Answer from the drawing. Dimensions are ordinates in mm from the lowest x, y and z of the part. A direction names the side the tool comes from. Coordinates: 2 decimals unless noted, no trailing zeros. Order: outer loops, then holes, each group sorted by start corner. A loop starts at its lowest first (then second) coordinate and runs counter-clockwise, first axis right, second up. Notation, with made-up numbers: (24.25, 87.5) -> (77.25, 87.5) arc R13 ccw to (77.25, 108.5) -> close; hole circle Ø2 at (20, -2). An arc over 180 degrees is marked (long way). Answer in a Markdown table with one row per item.
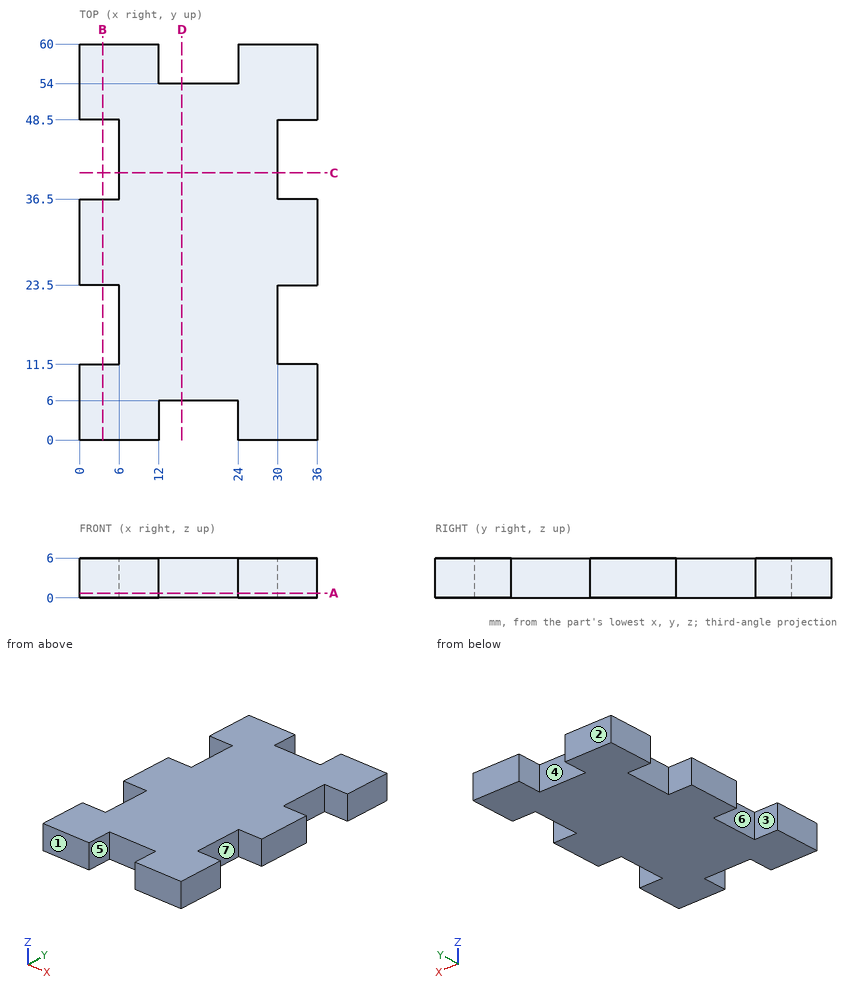
(1) Which of the six approach directions +Z, -Z, +X, -X, +Y, -Y give full straight-line access (tool end or side, diameter ignored) to the marked faces 4, 5, 6 and 7?
Check values:
| item | result |
|---|---|
| face 4 | +Z, -Z, +Y |
| face 5 | +Z, -Z, -Y |
| face 6 | +Z, -Z, -X |
| face 7 | +Z, -Z, +X |
(2) Find the intervals of material crossed by line 1 along Y through (x, z) = (31, 4.05); line 2 along X through (y, z) = (57, 1.9); line 3 along Y through (x, z) = (14, 3.95), in increasing order. Write a range as from..to.
Check values:
| item | result |
|---|---|
| line 1 | 0..11.5, 23.5..36.5, 48.5..60 |
| line 2 | 0..12, 24..36 |
| line 3 | 6..54 |
(3) A cutting plane is placed at A-A, the plane z = 0.7. Determine the outline of the cut face in (x, y).
Check values:
| item | result |
|---|---|
| outline | (0, 0) -> (12, 0) -> (12, 6) -> (24, 6) -> (24, 0) -> (36, 0) -> (36, 11.5) -> (30, 11.5) -> (30, 23.5) -> (36, 23.5) -> (36, 36.5) -> (30, 36.5) -> (30, 48.5) -> (36, 48.5) -> (36, 60) -> (24, 60) -> (24, 54) -> (12, 54) -> (12, 60) -> (0, 60) -> (0, 48.5) -> (6, 48.5) -> (6, 36.5) -> (0, 36.5) -> (0, 23.5) -> (6, 23.5) -> (6, 11.5) -> (0, 11.5) -> close |
(4) For a pull along Y with two mould halves and no side action, classify the marked faces 1, 2 and 3 as released by +Y, released by -Y, zero draft, split by the parting line, or undercut.
Check values:
| item | result |
|---|---|
| face 1 | released by -Y |
| face 2 | released by +Y |
| face 3 | undercut |
(5) A cutting plane is placed at B-B, the plane x = 3.5. Determine the outline of the cut face in (y, z).
Check values:
| item | result |
|---|---|
| outline | (0, 0) -> (11.5, 0) -> (11.5, 6) -> (0, 6) -> close; (23.5, 0) -> (36.5, 0) -> (36.5, 6) -> (23.5, 6) -> close; (48.5, 0) -> (60, 0) -> (60, 6) -> (48.5, 6) -> close |
(6) A cutting plane is placed at D-D, the plane x = 15.5. Determine the outline of the cut face in (y, z), then the cut area to 3 significant figures.
Check values:
| item | result |
|---|---|
| outline | (6, 0) -> (54, 0) -> (54, 6) -> (6, 6) -> close |
| area | 288 mm² |
(7) Flat-ended cylindrical pins translate along their axes: pin 1 (2 mm diameter, centred on x = 5.5, y = 18, fed in from +Z); pin 2 (1.8 mm diameter, centred on y = 17.5, z = 4.5, fed in from -X); pin 3 (3 mm diameter, centred on y = 14.5, z = 4, fed in from +X); pin 4 (2 mm diameter, centred on x = 22.5, z = 1, fed in from +Y). Find the tip coordinate at first contact, or state that the pin passes through.
Check values:
| item | result |
|---|---|
| pin 1 | z = 6 |
| pin 2 | x = 6 |
| pin 3 | x = 30 |
| pin 4 | y = 54 |
(8) A cutting plane is placed at C-C, the plane y = 40.5. Determine the outline of the cut face in (x, z), then the cut area to 3 significant figures.
Check values:
| item | result |
|---|---|
| outline | (6, 0) -> (30, 0) -> (30, 6) -> (6, 6) -> close |
| area | 144 mm² |
